Read the model definition and answer for the solid it produces. Units are mm, in the model's axes. Face numbers are marked on the shaded views. Coordinates: 2 decimals unless noted, no trailing zeros. Write each loop counter-clockwise with the first axis right and the second up, starting at its lowest first coordinate (ties: lowest second). Pieces come first, ordered by that corner, then holes.
(1) Section A-A on x = 0 is taken. Write down the section's boundary in (y, z), then the cut area to 3 significant figures.
(2) Given pin 1 (5 mm diameter, centred on x = 78.5, y = 9.5, fed in from +Z); pin 2 (4 mm diameter, centred on x = -48, y = 9, fed in from -Z); pin 3 (12 mm diameter, centred on y = -5, z = 71, fed in from +X), each flat-ended and moving along its own axis, determine where each tip first touches the part or whether it passes through.
(3) Section C-C on y = -6.5 is taken. Write down the section's boundary in (x, z).
(4) Section B-B on z = 0 is taken. Write down the section's boundary in (x, y).
(5) The mould has two halves that part along Y. Classify the marked faces 1 and 2: +Y half, -Y half, draft (parallel to the pull), parting line (faces both ways), or undercut.
(6) Section D-D on y = 14.5 is taken. Write down the section's boundary in (x, z).
(7) Find the intervals of material crossed by probe 1 along X at (y, z) = (-4, 0); probe 2 along X at (y, z) = (11, 0); probe 3 along Z at (x, y) = (13.5, 17.5), in increasing order.
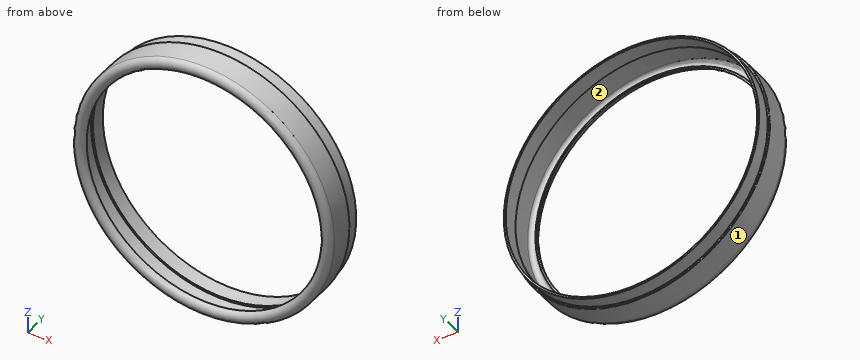
from build123d import *

# Parameters (mm, degrees)
FILLET1_R = 0.5


with BuildPart() as part:
    # Sketch1 → Revolve1 (revolve)
    with BuildSketch(Plane.YZ, mode=Mode.PRIVATE) as revolve1_sk:
        with BuildLine():
            Line((-9, 100), (9, 100))
            Line((9, 100), (9, 98.5))
            Line((9, 98.5), (19, 98.5))
            Line((19, 98.5), (19, 97))
            Line((19, 97), (7.5, 97))
            Line((7.5, 97), (7.5, 98.5))
            Line((7.5, 98.5), (-9, 98.5))
            ThreePointArc((-9, 98.5), (-12, 95.5), (-9, 92.5))
            Line((-9, 92.5), (-9, 91))
            ThreePointArc((-9, 91), (-13.5, 95.5), (-9, 100))
        make_face()
    revolve(revolve1_sk.sketch.rotate(Axis((0, -178.136934236, 0), (0, 1, 0)), 180), axis=Axis((0, -178.136934236, 0), (0, 1, 0)))

    # Fillet1
    fillet1_edges = [part.edges().sort_by_distance(p)[0] for p in [
        (0, 9, 100),
    ]]
    fillet(fillet1_edges, radius=FILLET1_R)


solid = part.part
Response:
1. outline: (-9, -100) - (8.5, -100) arc R0.5 ccw to (9, -99.5) - (9, -98.5) - (19, -98.5) - (19, -97) - (7.5, -97) - (7.5, -98.5) - (-9, -98.5) arc R3 cw to (-9, -92.5) - (-9, -91) arc R4.5 ccw to start; (-9, 91) - (-9, 92.5) arc R3 cw to (-9, 98.5) - (7.5, 98.5) - (7.5, 97) - (19, 97) - (19, 98.5) - (9, 98.5) - (9, 99.5) arc R0.5 ccw to (8.5, 100) - (-9, 100) arc R4.5 ccw to start
1. area: 124 mm2
2. pin 1: stops at z = 64.78
2. pin 2: stops at z = -88.76
2. pin 3: stops at x = 75.99
3. outline: circle Ø200 at (0, 0); hole circle Ø197 at (0, 0)
4. outline: (-100, -9) arc R4.5 ccw to (-91, -9) - (-92.5, -9) arc R3 cw to (-98.5, -9) - (-98.5, 7.5) - (-97, 7.5) - (-97, 19) - (-98.5, 19) - (-98.5, 9) - (-99.5, 9) arc R0.5 ccw to (-100, 8.5) - close; (91, -9) arc R4.5 ccw to (100, -9) - (100, 8.5) arc R0.5 ccw to (99.5, 9) - (98.5, 9) - (98.5, 19) - (97, 19) - (97, 7.5) - (98.5, 7.5) - (98.5, -9) arc R3 cw to (92.5, -9) - close
5. face 1: draft
5. face 2: undercut
6. outline: circle Ø197 at (0, 0); hole circle Ø194 at (0, 0)
7. probe 1: x = -100 to -98.5, 98.5 to 100
7. probe 2: x = -98.5 to -97, 97 to 98.5
7. probe 3: z = -97.57 to -96.06, 96.06 to 97.57
